Could you check a few things on this model? Use its own coordinates, in mm. A direction names the side the tool comes from. Give positions to 0.01 mm unless a question says otherwise; leave off trailing zeros. Loops run counter-clockwise (first coordinate to the right, second up) from the corner with the lowest first, then second, coordinate; pieces in that order, holes last.
1. Imagine slicing it at A-A (x = 0). List the corners of the cut face in (y, z) for me, plus the area to 3 significant figures.
2. Imagine slicing it at D-D (y = -4.25). List the corners of the cut face in (x, z) for me, plus the area to 3 significant figures.
3. Imagine slicing it at C-C (z = -41). List the corners of the cut face in (x, y) for me, plus the area to 3 significant figures.
4. For P1, Ø2.5, axis at x = -30.5, y = 13, coming from the -Z side; P2, Ø16, axis at x = -33.5, z = -11.5, coming from the -Y side; P3, Ø6, axis at y = 11.75, z = -51.25, coming from the +X side, each with a flat end and sliding along its axis, tell me the tip position at first contact or that it passes through.
5. Thinking about a two-plate mould opening in X: for faces 6 (the conical face through (-50.82, 11.26, -37.17)), 7 (the flat face through (-7, 10, 12.5)), 8 (the flat face through (10.5, 2, 0)), 9 (the conical face through (-60.82, 11.26, -37.17)), which applies, +X half, -X half, draft (parallel to the pull), parting line (faces both ways), or undercut?
6. Imagine slicing it at B-B (z = -51.25). List the corners of the cut face in (x, y) for me.
7. For faces 1 (the flat face through (-7.5, 6, 0)), 2 (the flat face through (-56.5, -7, -41)), 3 (the flat face through (-35, 12, -46.25)), 4 (the flat face through (-45.5, 12, -10)), 5 (the flat face through (-34, 7.75, -21)), which set-ups out of +Z, -Z, +X, -X, +Y, -Y let a thin tool reach every point of the face, with its end or its side?
8. I need wall thicknesses on line 1 along X through (y, z) = (11.25, -33.5); line 2 along Y through (x, z) = (-60.5, -30); line 3 along Y through (x, z) = (-50, -51.25). Which ranges of each line are inside material? Lowest first, please.
```python
from build123d import *

# Parameters (mm, degrees)
BOSS_EXTRUDE1_DEPTH            = 12.5
SKETCH2_W                      = 25
SKETCH2_H                      = 8
BOSS_EXTRUDE2_DEPTH            = 38
SKETCH7_W                      = 20
SKETCH7_H                      = 8
BOSS_EXTRUDE3_DEPTH            = 33.75
SKETCH10_W                     = 20
SKETCH10_H                     = 8
BOSS_EXTRUDE4_DEPTH            = 20
SKETCH11_W                     = 20
SKETCH11_H                     = 8
BOSS_EXTRUDE5_DEPTH            = 10
F_3_7_3_7_DIAMETER_HOLE2_D     = 3.7
F_3_7_3_7_DIAMETER_HOLE2_DEPTH = 10
F_3_7_3_7_DIAMETER_HOLE2_TIP   = 1.111592145
F_3_7_3_7_DIAMETER_HOLE1_D     = 3.7
F_3_7_3_7_DIAMETER_HOLE3_D     = 3.7
SKETCH12_W                     = 21
SKETCH12_H                     = 5.75
CUT_EXTRUDE1_DEPTH             = 88.763175649
SKETCH14_W                     = 4
SKETCH14_H                     = 30
BOSS_EXTRUDE7_DEPTH            = 15.5
SKETCH15_W                     = 30
SKETCH15_H                     = 2.25
BOSS_EXTRUDE8_DEPTH            = 5


with BuildPart() as part:
    # Sketch1 → Boss-Extrude1 (new, symmetric)
    with BuildSketch(Plane.XY):
        Polygon((-10.5, 0), (10.5, 0), (10.5, 3.5), (7.5, 3.5), (7.5, 15.75), (-7.5, 15.75), (-7.5, 3.5), (-10.5, 3.5), align=None)
    extrude(amount=BOSS_EXTRUDE1_DEPTH, both=True)

    # Sketch2 → Boss-Extrude2 (add)
    with BuildSketch(Plane.ZY.offset(7.5)):
        with Locations((0, 11.75)):
            Rectangle(SKETCH2_W, SKETCH2_H)
    extrude(amount=BOSS_EXTRUDE2_DEPTH)

    # Sketch7 → Boss-Extrude3 (add)
    with BuildSketch(Plane(origin=(0, 0, -12.5), x_dir=(-1, 0, 0), z_dir=(0, 0, -1))):
        with Locations((35.5, 11.75)):
            Rectangle(SKETCH7_W, SKETCH7_H)
    extrude(amount=BOSS_EXTRUDE3_DEPTH)

    # Sketch10 → Boss-Extrude4 (add)
    with BuildSketch(Plane.ZY.offset(45.5)):
        with Locations((-36.25, 11.75)):
            Rectangle(SKETCH10_W, SKETCH10_H)
    extrude(amount=BOSS_EXTRUDE4_DEPTH)

    # Sketch11 → Boss-Extrude5 (add)
    with BuildSketch(Plane(origin=(0, 0, -46.25), x_dir=(-1, 0, 0), z_dir=(0, 0, -1))):
        with Locations((55.5, 11.75)):
            Rectangle(SKETCH11_W, SKETCH11_H)
    extrude(amount=BOSS_EXTRUDE5_DEPTH)

    # Ø3.7 (3.7) Diameter Hole2
    with Locations(Plane.XY.offset(-26.25)):
        with Locations((-60.5, 11.25), (-50.5, 11.25)):
            Hole(F_3_7_3_7_DIAMETER_HOLE2_D / 2, depth=F_3_7_3_7_DIAMETER_HOLE2_DEPTH)
            with Locations((0, 0, -(F_3_7_3_7_DIAMETER_HOLE2_DEPTH + F_3_7_3_7_DIAMETER_HOLE2_TIP / 2))):  # 118° drill point
                Cone(0, F_3_7_3_7_DIAMETER_HOLE2_D / 2, F_3_7_3_7_DIAMETER_HOLE2_TIP, mode=Mode.SUBTRACT)

    # Ø3.7 (3.7) Diameter Hole1 (through all)
    with Locations(Plane.ZY.offset(65.5)):
        with Locations((-51.25, 11.75)):
            Hole(F_3_7_3_7_DIAMETER_HOLE1_D / 2)

    # Ø3.7 (3.7) Diameter Hole3 (through all)
    with Locations(Plane(origin=(0, 15.75, 0), x_dir=(1, 0, 0), z_dir=(0, 1, 0))):
        with Locations((0, 0)):
            Hole(F_3_7_3_7_DIAMETER_HOLE3_D / 2)

    # Sketch12 → Cut-Extrude1 (cut, through all)
    with BuildSketch(Plane(origin=(0, 15.75, 0), x_dir=(1, 0, 0), z_dir=(0, 1, 0))):
        with Locations((-35, -9.625)):
            Rectangle(SKETCH12_W, SKETCH12_H)
    extrude(amount=-CUT_EXTRUDE1_DEPTH, mode=Mode.SUBTRACT)

    # Sketch14 → Boss-Extrude7 (add)
    with BuildSketch(Plane.XZ.offset(-7.75)):
        with Locations((-63.5, -41.25)):
            Rectangle(SKETCH14_W, SKETCH14_H)
    extrude(amount=BOSS_EXTRUDE7_DEPTH)

    # Sketch15 → Boss-Extrude8 (add)
    with BuildSketch(Plane(origin=(-61.5, 0, 0), x_dir=(0, 0, -1), z_dir=(1, 0, 0))):
        with Locations((41.25, -6.625)):
            Rectangle(SKETCH15_W, SKETCH15_H)
    extrude(amount=BOSS_EXTRUDE8_DEPTH)


solid = part.part
```
Derived:
1. outline: (0, -12.5) - (15.75, -12.5) - (15.75, -1.85) - (0, -1.85) - close; (0, 1.85) - (15.75, 1.85) - (15.75, 12.5) - (0, 12.5) - close
1. area: 335 mm2
2. outline: (-65.5, -56.25) - (-61.5, -56.25) - (-61.5, -26.25) - (-65.5, -26.25) - close
2. area: 120 mm2
3. outline: (-65.5, -7.75) - (-56.5, -7.75) - (-56.5, -5.5) - (-61.5, -5.5) - (-61.5, 7.75) - (-25.5, 7.75) - (-25.5, 15.75) - (-65.5, 15.75) - close
3. area: 393 mm2
4. P1: stops at z = -46.25
4. P2: stops at y = 7.75
4. P3: stops at x = -45.5
5. face 6: undercut
5. face 7: draft
5. face 8: +X half
5. face 9: undercut
6. outline: (-65.5, -7.75) - (-56.5, -7.75) - (-56.5, -5.5) - (-61.5, -5.5) - (-61.5, 7.75) - (-45.5, 7.75) - (-45.5, 9.9) - (-65.5, 9.9) - close; (-65.5, 13.6) - (-45.5, 13.6) - (-45.5, 15.75) - (-65.5, 15.75) - close
7. face 1: +Z, -Z, -X
7. face 2: +Z, -Z, +X, -Y
7. face 3: -Z, +X, +Y, -Y
7. face 4: +Z, -X, +Y, -Y
7. face 5: +Z, -Z
8. line 1: x = -65.5 to -62.35, -58.65 to -52.35, -48.65 to -25.5
8. line 2: y = -7.75 to -5.5, 7.75 to 9.4, 13.1 to 15.75
8. line 3: y = 7.75 to 9.9, 13.6 to 15.75
